from build123d import *

# Parameters (mm, degrees)
F1_DEPTH = 76.2
F3_D     = 38.1


with BuildPart() as f1:
    # F0 (on Front) → F1 (new body)
    with BuildSketch(Plane.XZ):
        Polygon((0, 101.6), (0, 0), (38.1, 0), (38.1, 44.437758), (76.2, 44.437758), (76.2, 0), (127, 0), (127, 43.850472), (165.1, 43.850472), (165.1, 0), (203.2, 0), (203.2, 101.6), align=None)
    extrude(amount=-F1_DEPTH)

    # F3 (through all)
    with Locations(Plane.XY.offset(101.6)):
        with Locations((57.15, 38.1), (146.05, 38.1)):
            Hole(F3_D / 2)


solid = f1.part
Verification items for the finished model (mm, model axes). A direction names the side the tool comes from. Coordinates: 2 decimals unless noted, no trailing zeros. Write each loop counter-clockwise with the first axis right and the second up, starting at its lowest first coordinate (ties: lowest second). Pieces come first, ordered by that corner, then holes. Notation, with made-up numbers: (-23, 81.5) -> (20, 81.5) arc R30 cw to (20, 110.5) -> close; hole circle Ø7 at (9.5, 18.5). An arc over 180 degrees is marked (long way). One line per item, written item: value. Start each with the question number.
Q1. Go/stop test with flat-tipped pins: P1, Ø19, axis at x = 63, y = 64.5, coming from the -Z side; P2, Ø5, axis at x = 158.5, y = 49.5, coming from the -Z side. Record where each tip stops, or that it passes through.
Q2. Cross-section at B-B on z = 9. Enter the section's corners in (x, y).
Q3. Cross-section at A-A on x = 146.05. Enter the section's corners in (y, z), and give its area (3 significant figures).
Q4. Access from +Z, -Z, +X, -X, +Y, -Y to the whole of each face (thin tool, end or side, straight path). Record for faces 1 (the flat face through (57, 65, 44.438)), 2 (the flat face through (184, 38, 0)).
Q5. Thickness scan on L1, parallel to X at y = 38, z = 88; L2, parallel to Y at x = 57.15, z = 72; L3, parallel to X at y = 49, z = 58. Record the ranges inside material, lowest first. Write a range as from..to.
Q6. Cross-section at C-C on z = 68.5. Enter the section's corners in (x, y), and give its area (3 significant figures).
Q7. Cross-section at D-D on y = 25.5. Enter the section's corners in (x, z).
Q8. Mould release check, pull along Y, two halves, no side actions. Record for faces 3 (the cylindrical face through (39.553, 30.804, 72.619)), 4 (the flat face through (0, 38, 52)), 5 (the flat face through (100, 76.2, 52)): pulls with the +Y half, pulls with the -Y half, needs draft (parallel to the pull), parting line crosses it, or undercut.
Checked values:
1. P1: stops at z = 44.44
1. P2: stops at z = 43.85
2. outline: (0, 0) -> (38.1, 0) -> (38.1, 76.2) -> (0, 76.2) -> close; (76.2, 0) -> (127, 0) -> (127, 76.2) -> (76.2, 76.2) -> close; (165.1, 0) -> (203.2, 0) -> (203.2, 76.2) -> (165.1, 76.2) -> close
3. outline: (0, 43.85) -> (19.05, 43.85) -> (19.05, 101.6) -> (0, 101.6) -> close; (57.15, 43.85) -> (76.2, 43.85) -> (76.2, 101.6) -> (57.15, 101.6) -> close
3. area: 2,200 mm²
4. face 1: -Z, +Y, -Y
4. face 2: -Z, +X, -X, +Y, -Y
5. L1: x = 0..38.1, 76.2..127, 165.1..203.2
5. L2: y = 0..19.05, 57.15..76.2
5. L3: x = 0..41.53, 72.77..130.43, 161.67..203.2
6. outline: (0, 0) -> (203.2, 0) -> (203.2, 76.2) -> (0, 76.2) -> close; hole circle Ø38.1 at (57.15, 38.1); hole circle Ø38.1 at (146.05, 38.1)
6. area: 13,200 mm²
7. outline: (0, 0) -> (38.1, 0) -> (38.1, 44.44) -> (42.86, 44.44) -> (42.86, 101.6) -> (0, 101.6) -> close; (71.44, 44.44) -> (76.2, 44.44) -> (76.2, 0) -> (127, 0) -> (127, 43.85) -> (131.76, 43.85) -> (131.76, 101.6) -> (71.44, 101.6) -> close; (160.34, 43.85) -> (165.1, 43.85) -> (165.1, 0) -> (203.2, 0) -> (203.2, 101.6) -> (160.34, 101.6) -> close
8. face 3: undercut
8. face 4: needs draft
8. face 5: pulls with the +Y half
